```python
from build123d import *

# Parameters (mm, degrees)
F0_R     = 30
F0_R_2   = 25
F1_DEPTH = 40
F3_DEPTH = 52.8


with BuildPart() as f1:
    # F0 (on Top) → F1 (new body, symmetric)
    with BuildSketch(Plane.XY):
        Circle(F0_R)
        Circle(F0_R_2, mode=Mode.SUBTRACT)
    extrude(amount=F1_DEPTH, both=True)

    # F2 (on Front) → F3 (cut, symmetric)
    with BuildSketch(Plane.XZ):
        Polygon((7.5, 40), (-7.5, 40), (-7.5, 20), (-15, 20), (-15, 0), (15, 0), (15, 20), (7.5, 20), align=None)
    extrude(amount=F3_DEPTH, both=True, mode=Mode.SUBTRACT)


solid = f1.part
```
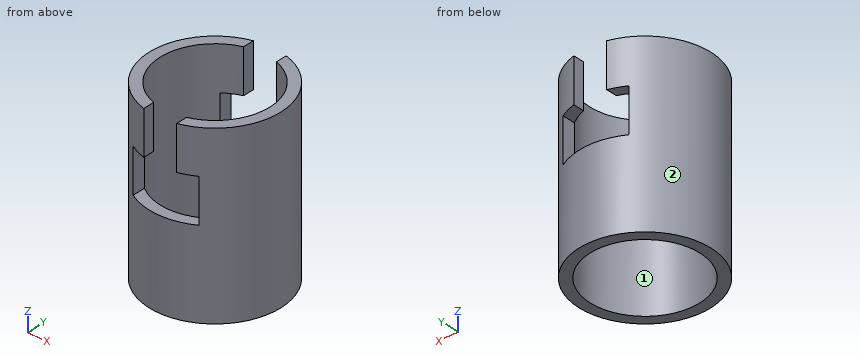
Geometry: final body of the model. Coordinates: model frame, mm. Face numbers are marked on the shaded views. Coordinates: 2 decimals unless noted, no trailing zeros. Order: outer loops, then holes, each group sorted by start corner. A loop starts at its lowest first (then second) coordinate and runs counter-clockwise, first axis right, second up. Notation, with made-up numbers: (32, -11) - (81, -11) arc R8 ccw to (81, 0) - close; hole circle Ø11 at (67.5, -9). An arc over 180 degrees is marked (long way). Return JSON: item names as keys, results as strings. Group by question number.
1. Material intervals for line 1 along Z through (x, y) = (-8.5, 26); line 2 along Y through (x, z) = (18, 26.5); line 3 along X through (y, z) = (27.5, 25.5), sorted ascending. Write a range as [from, to].
2. Pin query (flat end, axial travel): pin 1 (6 mm diameter, centred on y = 15.5, z = -28.5, fed in from -X); pin 2 (5 mm diameter, centred on y = -22, z = 6, fed in from -X); pin 3 (12 mm diameter, centred on y = 9, z = 16, fed in from -X); pin 4 (6 mm diameter, centred on x = -23.5, y = 6, fed in from +Z). Return the tip coordinate at first contact, or that it passes through.
3. Cut plane A-A (z = 1). Output: boundary loops of the cut face in (x, y), plus the area to 3 significant figures.
4. Pull-direction query (X, two-part tool) for the marked faces 1 and 2; classes: pulls with the +X half, pulls with the -X half, needs draft (parallel to the pull), parting line crosses it, or undercut.
5. Cut plane C-C (z = -29). Output: boundary loops of the cut face in (x, y).
6. Cut plane B-B (x = 0). Output: boundary loops of the cut face in (y, z).
Resolved:
{
 "1": {"line 1": "z = [-40, 0], [20, 40]", "line 2": "y = [-24, -17.35], [17.35, 24]", "line 3": "x = [-11.99, -7.5], [7.5, 11.99]"},
 "2": {"pin 1": "stops at x = -27.27", "pin 2": "stops at x = -22.8", "pin 3": "stops at x = -29.85", "pin 4": "stops at z = 40"},
 "3": {"outline": "(-15, -25.98) - (-15, -20) arc R25 cw to (-15, 20) - (-15, 25.98) arc R30 ccw to start; (15, -25.98) arc R30 ccw to (15, 25.98) - (15, 20) arc R25 cw to (15, -20) - close", "area": "546 mm²"},
 "4": {"face 1": "undercut", "face 2": "parting line crosses it"},
 "5": {"outline": "circle Ø60 at (0, 0); hole circle Ø50 at (0, 0)"},
 "6": {"outline": "(-30, -40) - (-25, -40) - (-25, 0) - (-30, 0) - close; (25, -40) - (30, -40) - (30, 0) - (25, 0) - close"}
}
